Part model, mm, in its own coordinate system. A direction names the side the tool comes from. Give positions to 0.01 mm unless a question says otherwise; leave off trailing zeros. Order: outer loops, then holes, each group sorted by start corner. A loop starts at its lowest first (then second) coordinate and runs counter-clockwise, first axis right, second up. Notation, with made-up numbers: M 21.5,22 L 41.5,22 A11 cw 41.5,30 Z; hole C 83.25,69.25 d11. An arc over 180 degrees is marked long. Return JSON: item names as keys, results as strings.
from build123d import *

# Parameters (mm, degrees)
SKETCH1_W           = 36.195
SKETCH1_H           = 31.027347648
SKETCH1_R           = 3.2639
BOSS_EXTRUDE1_DEPTH = 7.10692
BOSS_EXTRUDE3_DEPTH = 6.35
FILLET1_R           = 2.54


with BuildPart() as part:
    # Sketch1 → Boss-Extrude1 (new body)
    with BuildSketch(Plane.XY):
        with Locations((-48.5775, -7.089116399)):
            Rectangle(SKETCH1_W, SKETCH1_H)
        with Locations((-51.577868645, -7.089116399)):
            Circle(SKETCH1_R, mode=Mode.SUBTRACT)
    extrude(amount=BOSS_EXTRUDE1_DEPTH)

    # Sketch2 → Boss-Extrude3 (add)
    with BuildSketch(Plane(origin=(0, 0, 0), x_dir=(-1, 0, 0), z_dir=(0, 0, -1))):
        Polygon((30.48, -19.681790223), (30.48, -22.602790223), (66.675, -22.602790223), (66.675, 8.424557425), (30.48, 8.424557425), (30.48, 5.503557425), (63.754, 5.503557425), (63.754, -19.681790223), align=None)
    extrude(amount=BOSS_EXTRUDE3_DEPTH)

    # Fillet1
    fillet1_edges = [part.edges().sort_by_distance(p)[0] for p in [
        (-48.5775, 8.424557425, -6.35),
        (-66.675, -7.089116399, -6.35),
        (-48.5775, -22.602790223, -6.35),
        (-66.675, 8.424557425, 0.37846),
        (-30.48, 8.424557425, 0.37846),
        (-30.48, -22.602790223, 0.37846),
        (-66.675, -22.602790223, 0.37846),
    ]]
    fillet(fillet1_edges, radius=FILLET1_R)


solid = part.part
Q1. Band-saw the part on D-D (y = -15). Give the cut face in (x, z) (3 decimals).
Established:
{"outline": "M -66.675,-3.81 A2.54 ccw -64.135,-6.35 L -63.754,-6.35 L -63.754,0 L -30.48,0 L -30.48,7.107 L -66.675,7.107 Z"}
Q2. Band-saw the part on B-B (y = -6). Give the cut face in (x, z) (3 decimals).
Established:
{"outline": "M -66.675,-3.81 A2.54 ccw -64.135,-6.35 L -63.754,-6.35 L -63.754,0 L -54.655,0 L -54.655,7.107 L -66.675,7.107 Z; M -48.501,0 L -30.48,0 L -30.48,7.107 L -48.501,7.107 Z"}
Q3. Band-saw the part on A-A (z = 1.25). Give the cut face in (x, y) (3 decimals).
Established:
{"outline": "M -66.675,-20.063 A2.54 ccw -64.135,-22.603 L -33.02,-22.603 A2.54 ccw -30.48,-20.063 L -30.48,5.885 A2.54 ccw -33.02,8.425 L -64.135,8.425 A2.54 ccw -66.675,5.885 Z; hole C -51.578,-7.089 d6.528"}
Q4. Pin check, flat tips, straight feed: pin 1 (1.9 mm diameter, centred on x = -42, z = -4, fed in from -Y); pin 2 (3 mm diameter, centred on y = -13, z = -4, fed in from +X); pin 3 (7.5 mm diameter, centred on x = -48, y = -1, fed in from -Z). Stop position of each tip, or through.
Established:
{"pin 1": "stops at y = -22.6", "pin 2": "stops at x = -63.75", "pin 3": "stops at z = 0"}
Q5. 3-axis set-ups, long thin cutter, end or side, ignore diameter. For faces 4 (the flat face through (-48, -22.603, 2)), 5 (the flat face through (-63.754, -7, -3)): which of +Z, -Z, +X, -X, +Y, -Y reach the whole face in a straight line?
Established:
{"face 4": "+Z, -Z, +X, -X, -Y", "face 5": "-Z, +X"}
Q6. Band-saw the part on C-C (x = -47). Give the cut face in (y, z).
Established:
{"outline": "M -22.6,-3.81 A2.54 ccw -20.06,-6.35 L -19.68,-6.35 L -19.68,0 L 5.5,0 L 5.5,-6.35 L 5.88,-6.35 A2.54 ccw 8.42,-3.81 L 8.42,7.11 L -22.6,7.11 Z"}
Q7. Two-plate mould, pull along Y, no slides. Class faces 1 (the cylindrical face through (-47.072, 7.7, -5.586)), 2 (the flat face through (-47, -7, 0)), 3 (the cylindrical face through (-65.95, -21.84, 1.57)): +Y half, -Y half, draft (parallel to the pull), parting line (faces both ways), or undercut.
Established:
{"face 1": "+Y half", "face 2": "undercut", "face 3": "-Y half"}
Q8. Probe line 1 along Y through (x, z) = (-37, -0.5); line 2 along Z through (x, y) = (-41, -5); line 3 along X through (y, z) = (-7, 3) (3 decimals). List the from-to ranges inside material, lowest first.
Established:
{"line 1": "y = -22.6 to -19.68, 5.5 to 8.42", "line 2": "z = 0 to 7.11", "line 3": "x = -66.675 to -54.841, -48.315 to -30.48"}
